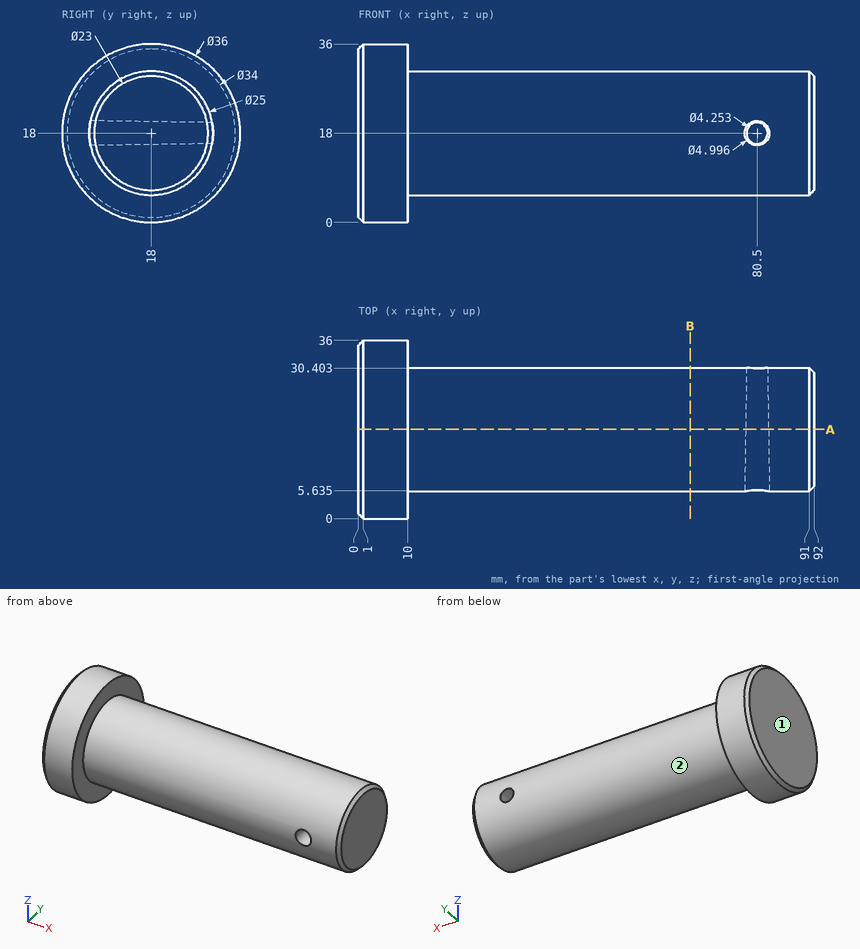
Print and shaded views of the part. All mm, measured from the part's lowest x, y and z. A direction names the side the tool comes from. Coordinates: 2 decimals unless noted, no trailing zeros. Order: outer loops, then holes, each group sorted by start corner. A loop starts at its lowest first (then second) coordinate and runs counter-clockwise, first axis right, second up. Notation, with made-up numbers: (56, 83.25) -> (91, 83.25) arc R23 cw to (91, 105.25) -> close; hole circle Ø9 at (-32.75, -2). An arc over 180 degrees is marked (long way). Use one line per item in the form item = value. Start each with the question number.
1) Band-saw the part on A-A on y = 18. Give the cut face in (x, z) (1 decimal), then the cut area to 3 significant figures.
2) Band-saw the part on B-B on x = 67. Give the cut face in (y, z).
3) Drop flat-ended pins along their axis: pin 1 (1 mm diameter, centred on x = 44, z = 29, fed in from +Y) (1 decimal); pin 2 (8 mm diameter, centred on y = 30, z = 32, fed in from +X); pin 3 (2 mm diameter, centred on x = 73.5, z = 24, fed in from +Y). Give the stop position or say it passes through.
4) Tool access for the marked faces 1 and 2: list every direction of +Z, -Z, +X, -X, +Y, -Y with a clear straight run to the whole face (end or side of a thin tool).
5) Drill centre lines: L1, parallel to X at y = 20.5, z = 33.5; L2, parallel to X at y = 18.5, z = 17 (1 decimal); L3, parallel to Z at x = 59, y = 13 (1 decimal). Where is each one in solid material? Low to high. Write a range as [from, to].
Entries:
q1.outline = (0, 1) -> (1, 0) -> (10, 0) -> (10, 5.5) -> (91, 5.5) -> (92, 6.5) -> (92, 29.5) -> (91, 30.5) -> (10, 30.5) -> (10, 36) -> (1, 36) -> (0, 35) -> close; hole circle Ø4.6 at (80.5, 18)
q1.area = 2,390 mm2
q2.outline = circle Ø25 at (18, 18)
q3.pin_1 = 24.8
q3.pin_2 = 10
q3.pin_3 = 29.46
q4.face_1 = +Z, -Z, -X, +Y, -Y
q4.face_2 = +X
q5.L1 = [0, 10]
q5.L2 = [0, 78.4], [82.6, 92]
q5.L3 = [6.5, 29.5]
